For this review, use the dimensioned drawing (mm, ordinates from the lowest corner) and the shaded views. A direction names the side the tool comes from. Round coordinates to 2 decimals unless told otherwise and drop trailing zeros. Write each loop counter-clockwise with the first axis right and the second up, starting at its lowest first coordinate (ties: lowest second). Pieces come first, ordered by that corner, then holes. Notation, with made-up numbers: (82.25, 84) -> (128.25, 84) arc R13 ccw to (128.25, 92) -> close; hole circle Ø10 at (51, -30). An arc over 180 degrees is marked (long way). Answer as CSV lines item,"result". Start each with the question number.
Item 1: Take a section at D-D on y = 1. Give the boundary of the cut face in (x, z).
Item 2: For pin 1 Ø5 at (x, z) = (9.5, 6) entering from +Y; pin 2 Ø1 at (x, z) = (7, 10) entering from -Y; pin 3 Ø5 at (x, z) = (2, 9) entering from -Y, all flat-tipped, find the tip position at first contact; note any pin that passes through.
Item 3: Machinability: for the marked faces 1 and 2, which of the approach directions +Z, -Z, +X, -X, +Y, -Y give a long, thin tool a straight path to every point of the face, cutting with its end or side? Answer none if there is none.
Item 4: Mouldability with a two-part tool opening along Z and no side actions: class the marked faces 3, 4 and 5 as +Z half, -Z half, draft (parallel to the pull), parting line (faces both ways), or undercut.
Item 5: Take a section at A-A on z = 6. Give the boundary of the cut face in (x, y) (3 decimals), then the cut area to 3 significant figures.
Item 6: Take a section at C-C on x = 7. Give the boundary of the cut face in (y, z) (3 decimals).
Item 7: Wall thickness on probe 1 along Z at (x, y) = (8.25, 6) (3 decimals); probe 2 along X at (y, z) = (9.25, 9.75); probe 3 along Z at (x, y) = (3.75, 4.5): over which ranges is each line inside the solid? List them lowest first. Write a range as from..to.
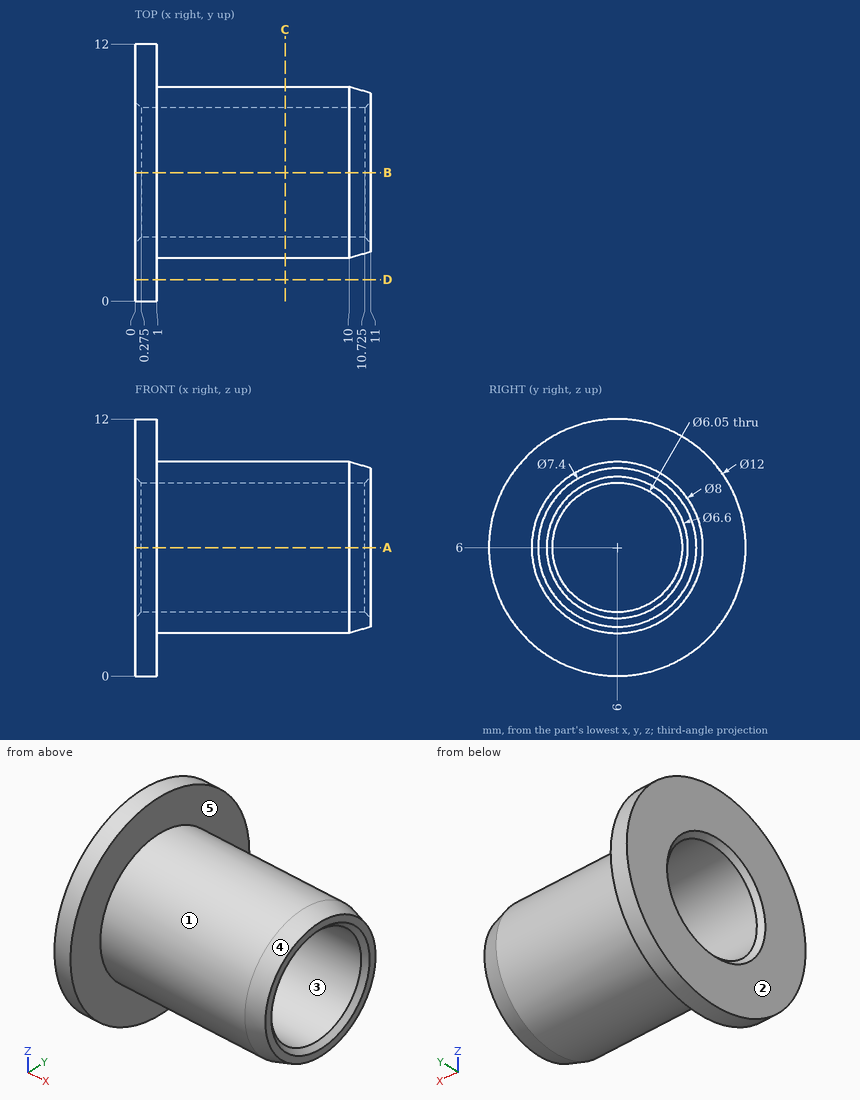
Output values:
1,outline,"(0, 2.68) -> (1, 2.68) -> (1, 9.32) -> (0, 9.32) -> close"
2,pin 1,"stops at y = 10"
2,pin 2,"stops at y = 4.06"
2,pin 3,"stops at y = 0.04"
3,face 1,"+X"
3,face 2,"+Z, -Z, -X, +Y, -Y"
4,face 3,"undercut"
4,face 4,"parting line"
4,face 5,"draft"
5,outline,"(0, 0) -> (1, 0) -> (1, 2) -> (10, 2) -> (11, 2.3) -> (11, 2.7) -> (10.725, 2.975) -> (0.275, 2.975) -> (0, 2.7) -> close; (0, 9.3) -> (0.275, 9.025) -> (10.725, 9.025) -> (11, 9.3) -> (11, 9.7) -> (10, 10) -> (1, 10) -> (1, 12) -> (0, 12) -> close"
5,area,"25.0 mm^2"
6,outline,"circle Ø8 at (6, 6); hole circle Ø6.05 at (6, 6)"
7,probe 1,"z = 2..2.975, 9.025..10"
7,probe 2,"x = 0..1"
7,probe 3,"z = 2.29..3.37, 8.63..9.71"
